```python
from build123d import *

# Parameters (mm, degrees)
SKETCH1_R                   = 6.35
SKETCH1_R_2                 = 3.3655
BOSS_EXTRUDE1_DEPTH         = 82.55
F_3_8_16_TAPPED_HOLE0_D     = 7.9375
F_3_8_16_TAPPED_HOLE0_DEPTH = 19.05
F_3_8_16_TAPPED_HOLE0_TIP   = 2.384665582
CUT_EXTRUDE2_DEPTH          = 7.35
SKETCH75_W                  = 12.7
SKETCH75_H                  = 5.318125
CUT_REVOLVE1_ANGLE          = 45
CUT_EXTRUDE3_DEPTH          = 9.980256262
F_3_8_16_TAPPED_HOLE1_D     = 7.9375
F_3_8_16_TAPPED_HOLE1_DEPTH = 19.05
F_3_8_16_TAPPED_HOLE1_TIP   = 2.384665582


with BuildPart() as part:
    # Sketch1 → Boss-Extrude1 (new body)
    with BuildSketch(Plane.XY):
        Circle(SKETCH1_R)
        Circle(SKETCH1_R_2, mode=Mode.SUBTRACT)
    extrude(amount=BOSS_EXTRUDE1_DEPTH)

    # 3/8-16 Tapped Hole0
    with Locations(Plane(origin=(0, 0, 0), x_dir=(-1, 0, 0), z_dir=(0, 0, -1))):
        with Locations((0, 0)):
            Hole(F_3_8_16_TAPPED_HOLE0_D / 2, depth=F_3_8_16_TAPPED_HOLE0_DEPTH)
            with Locations((0, 0, -(F_3_8_16_TAPPED_HOLE0_DEPTH + F_3_8_16_TAPPED_HOLE0_TIP / 2))):  # 118° drill point
                Cone(0, F_3_8_16_TAPPED_HOLE0_D / 2, F_3_8_16_TAPPED_HOLE0_TIP, mode=Mode.SUBTRACT)

    # Sketch13 → Cut-Extrude2 (cut, through all)
    with BuildSketch(Plane(origin=(0, 0, 0), x_dir=(0, 0, -1), z_dir=(1, 0, 0))):
        with BuildLine():
            Line((-49.53, 2.778125), (-46.99, 2.778125))
            ThreePointArc((-46.99, 2.778125), (-44.211875, 0), (-46.99, -2.778125))
            Line((-46.99, -2.778125), (-49.53, -2.778125))
            ThreePointArc((-49.53, -2.778125), (-52.308125, 0), (-49.53, 2.778125))
        make_face()
    extrude(amount=CUT_EXTRUDE2_DEPTH, mode=Mode.SUBTRACT)

    # Sketch75 → Cut-Revolve1 (revolve, cut)
    with BuildSketch(Plane(origin=(0, 0, 0), x_dir=(1, 0, 0), z_dir=(0, 1, 0))):
        with Locations((6.35, -46.8709375)):
            Rectangle(SKETCH75_W, SKETCH75_H)
    revolve(axis=Axis((0, 0, 0), (0, 0, 1)), revolution_arc=CUT_REVOLVE1_ANGLE, mode=Mode.SUBTRACT)

    # Sketch52 → Cut-Extrude3 (cut, through all)
    with BuildSketch(Plane(origin=(0, 0, 0), x_dir=(0.707106781, -0.707106781, 0), z_dir=(0.707106781, 0.707106781, 0))):
        with BuildLine():
            Line((-2.778125, -55.88), (-2.778125, -46.99))
            ThreePointArc((-2.778125, -46.99), (0, -44.211875), (2.778125, -46.99))
            Line((2.778125, -46.99), (2.778125, -55.88))
            ThreePointArc((2.778125, -55.88), (0, -58.658125), (-2.778125, -55.88))
        make_face()
    extrude(amount=CUT_EXTRUDE3_DEPTH, mode=Mode.SUBTRACT)

    # 3/8-16 Tapped Hole1
    with Locations(Plane.XY.offset(82.55)):
        with Locations((0, 0)):
            Hole(F_3_8_16_TAPPED_HOLE1_D / 2, depth=F_3_8_16_TAPPED_HOLE1_DEPTH)
            with Locations((0, 0, -(F_3_8_16_TAPPED_HOLE1_DEPTH + F_3_8_16_TAPPED_HOLE1_TIP / 2))):  # 118° drill point
                Cone(0, F_3_8_16_TAPPED_HOLE1_D / 2, F_3_8_16_TAPPED_HOLE1_TIP, mode=Mode.SUBTRACT)


solid = part.part
```
Here's how the part is built. I have some questions about the finished solid (model axes, mm). A direction names the side the tool comes from. Give positions to 0.01 mm unless a question says otherwise; leave off trailing zeros. Loops run counter-clockwise (first coordinate to the right, second up) from the corner with the lowest first, then second, coordinate; pieces in that order, holes last. Notation, with made-up numbers: M -22.5,88 L -14.5,88 A19 ccw -14.5,102 Z; hole C -13.75,-21 d8. An arc over 180 degrees is marked long. Put each result on its own line as item: value. Start each with the question number.
(1) Will these pins go through, and if not, where does the flat tip stop? pin 1 Ø7 at (x, y) = (0, 0) entering from +Z; pin 2 Ø2 at (x, z) = (-4, 66) entering from +Y; pin 3 Ø3 at (x, z) = (4, 48.5) entering from +Y.
(2) I need wall thicknesses on line 1 along Y through (x, z) = (0, 34); line 2 along Y through (x, z) = (0, 75); line 3 along Z through (x, y) = (3, 5). Which ranges of each line are inside material? Lowest first, please. Write a range as [from, to].
(3) For faces 5 (the cylindrical face through (4.588, -1.68, 51.743)), 6 (the cylindrical face through (3.288, 3.201, 58.657)), 7 (the flat face through (4.64, 0.71, 54.1)), which set-ups out of +Z, -Z, +X, -X, +Y, -Y let a thin tool reach every point of the face, with its end or its side?
(4) If we mould it in two halves opening along Y, with no side actions, what happens to faces 1 (the flat face through (3, 3, 82.55)), 2 (the flat face through (0.71, 4.64, 51.5)), 3 (the cylindrical face through (-5.04, -3.86, 40.7)), 4 (the cylindrical face through (-0.86, -3.874, 9.658))? For each: +Y half, -Y half, draft (parallel to the pull), parting line (faces both ways), or undercut.
(5) I want a section at A-A on z = 42. Please give me the cut outline in (x, y), then the cut area to 3 significant figures.
Answer block:
1. pin 1: z = 63.22
1. pin 2: y = 5.6
1. pin 3: y = -2.74
2. line 1: [-6.35, -3.37], [3.37, 6.35]
2. line 2: [-6.35, -3.97], [3.97, 6.35]
2. line 3: [0, 44.6], [58.27, 82.55]
3. face 5: +X
3. face 6: none
3. face 7: +Y
4. face 1: draft
4. face 2: undercut
4. face 3: parting line
4. face 4: undercut
5. outline: C 0,0 d12.7; hole C 0,0 d6.73
5. area: 91.1 mm^2
